```python
from build123d import *

# Parameters (mm, degrees)
SKETCH1_R           = 2.54
SKETCH1_R_2         = 14.2748
BOSS_EXTRUDE1_DEPTH = 12.7
CUT_EXTRUDE2_DEPTH  = 13.7
SKETCH3_R           = 2.4765
CUT_EXTRUDE3_DEPTH  = 13.7


with BuildPart() as part:
    # Sketch1 → Boss-Extrude1 (new body)
    with BuildSketch(Plane(origin=(0, 0, 0), x_dir=(1, 0, 0), z_dir=(0, 1, 0))):
        Polygon((152.4, 133.35), (-152.4, 133.35), (-152.4, -57.15), (-88.9, -57.15), (88.9, -57.15), (152.4, -57.15), align=None)
        with Locations((-114.3, 61.722)):
            Circle(SKETCH1_R, mode=Mode.SUBTRACT)
        with Locations((-114.3, 87.122)):
            Circle(SKETCH1_R_2, mode=Mode.SUBTRACT)
        with Locations((-114.3, 112.522)):
            Circle(SKETCH1_R, mode=Mode.SUBTRACT)
        with Locations((114.3, 61.722)):
            Circle(SKETCH1_R, mode=Mode.SUBTRACT)
        with Locations((114.3, 87.122)):
            Circle(SKETCH1_R_2, mode=Mode.SUBTRACT)
        with Locations((114.3, 112.522)):
            Circle(SKETCH1_R, mode=Mode.SUBTRACT)
    extrude(amount=BOSS_EXTRUDE1_DEPTH)

    # Sketch2 → Cut-Extrude2 (cut, through all)
    with BuildSketch(Plane(origin=(0, 12.7, 0), x_dir=(1, 0, 0), z_dir=(0, 1, 0))):
        with BuildLine():
            Line((108.5453125, -25.4), (108.5453125, 12.7))
            ThreePointArc((108.5453125, 12.7), (111.125, 15.2796875), (113.7046875, 12.7))
            Line((113.7046875, 12.7), (113.7046875, -25.4))
            ThreePointArc((113.7046875, -25.4), (111.125, -27.9796875), (108.5453125, -25.4))
        make_face()
        with BuildLine():
            Line((140.2953125, -25.4), (140.2953125, 12.7))
            ThreePointArc((140.2953125, 12.7), (142.875, 15.2796875), (145.4546875, 12.7))
            Line((145.4546875, 12.7), (145.4546875, -25.4))
            ThreePointArc((145.4546875, -25.4), (142.875, -27.9796875), (140.2953125, -25.4))
        make_face()
    extrude(amount=-CUT_EXTRUDE2_DEPTH, mode=Mode.SUBTRACT)

    # Sketch3 → Cut-Extrude3 (cut, through all)
    with BuildSketch(Plane(origin=(0, 0, 0), x_dir=(-1, 0, 0), z_dir=(0, -1, 0))):
        with Locations((-111.125, -44.45)):
            Circle(SKETCH3_R)
        with Locations((-111.125, 31.75)):
            Circle(SKETCH3_R)
        with Locations((111.125, 31.75)):
            Circle(SKETCH3_R)
        with Locations((111.125, -44.45)):
            Circle(SKETCH3_R)
    extrude(amount=-CUT_EXTRUDE3_DEPTH, mode=Mode.SUBTRACT)


solid = part.part
```
Could you check a few things on this model? Use its own coordinates, in mm. A direction names the side the tool comes from. Round coordinates to 2 decimals unless told otherwise and drop trailing zeros. Answer in a Markdown table with one row per item. Add a question column.
Q1. If we mould it in two halves opening along X, with no side actions, what happens to faces 1 (the flat face through (-2, 0, -39)), 2 (the flat face through (-152.4, 6, -39)), 3 (the flat face through (145.455, 6, 6))? For each: +X half, -X half, draft (parallel to the pull), parting line (faces both ways), or undercut.
Q2. Imagine slicing it at A-A (y = 10.5). Give the number of separate pieces and of enclosed holes in the cut face, then the cut area to 3 significant figures.
Q3. If I drill on line 1 (X direction, y = 5.5, z = 44.45); line 2 (X direction, y = 3.25, z = -1); line 3 (Z direction, x = 114.3, y = 4.5), over which ranges is the centre line in solid material (lowest first)? Write a range as from..to.
Q4. On a 3-axis mill with a long thin cutter (end or side, diameter ignored), from which of +Z, -Z, +X, -X, +Y, -Y can I reach the whole of each face in a straight line? I mean faces 4 (the flat face through (108.545, 6, 7)), 5 (the flat face through (152.4, 6, -37)). Say none if no direction works.
Values:
| question | item | result |
|---|---|---|
| 1 | face 1 | draft |
| 1 | face 2 | -X half |
| 1 | face 3 | undercut |
| 2 | separate pieces | 1 |
| 2 | enclosed holes | 12 |
| 2 | area | 56,200 mm^2 |
| 3 | line 1 | -152.4..-113.6, -108.65..108.65, 113.6..152.4 |
| 3 | line 2 | -152.4..108.55, 113.7..140.3, 145.45..152.4 |
| 3 | line 3 | -133.35..-115.06, -109.98..-101.4, -72.85..-64.26, -59.18..57.15 |
| 4 | face 4 | +Y, -Y |
| 4 | face 5 | +Z, -Z, +X, +Y, -Y |
